Source: CAD feature listing. Evaluate the final solid. Frame: model axes, mm. Coordinates: 2 decimals unless noted, no trailing zeros. Order: outer loops, then holes, each group sorted by start corner. A loop starts at its lowest first (then second) coordinate and runs counter-clockwise, first axis right, second up.
Item 1: Mould query, pull axis Y, two halves, no side actions, for faces 1 (the flat face through (-41, 49, 1.6)), 2 (the cylindrical face through (5.533, 4.807, 0.789)), 3 (the cylindrical face through (-77.7, 84.3, 0.8)). Classes: released by +Y, released by -Y, zero draft, split by the parting line, or undercut.
Item 2: Section A-A on z = 1.05. Return the cut outline in (x, y), then the cut area to 3 significant figures.
Item 3: Ray query, line 1 (X direction, y = 8, z = 1.1); line 2 (Y direction, x = -2, z = 1.4); line 3 (Y direction, x = -69, z = 0.85). Return the intervals inside material, ascending.
Item 4: Section B-B on x = -70.5. Return the cut outline in (y, z), then the cut area to 3 significant figures.
Item 5: Contact query for flat-ended pins moving along their axis: P1, Ø0.8, axis at y = 91, z = 0.5, coming from the -X side; P2, Ø0.8, axis at x = -79, z = 0.5, coming from the +Y side. Output: stop coordinate, or through.
from build123d import *

# Parameters (mm, degrees)
BOSS_EXTRUDE1_DEPTH        = 1.6
F_3_2_3_2_DIAMETER_HOLE3_D = 3.2


with BuildPart() as part:
    # Sketch1 → Boss-Extrude1 (new body)
    with BuildSketch(Plane.XY):
        with BuildLine():
            Line((-87.56534388, 82.95185693), (-87.56534388, 6.95185693))
            ThreePointArc((-87.56534388, 6.95185693), (-86.686664224, 4.830536587), (-84.56534388, 3.95185693))
            Line((-84.56534388, 3.95185693), (3.43465612, 3.95185693))
            ThreePointArc((3.43465612, 3.95185693), (5.555976464, 4.830536587), (6.43465612, 6.95185693))
            Line((6.43465612, 6.95185693), (6.43465612, 88.95185693))
            ThreePointArc((6.43465612, 88.95185693), (5.555976464, 91.073177274), (3.43465612, 91.95185693))
            Line((3.43465612, 91.95185693), (0.93465612, 91.95185693))
            Line((0.93465612, 91.95185693), (-64.56534388, 91.95185693))
            Line((-64.56534388, 91.95185693), (-64.56534388, 87.95185693))
            ThreePointArc((-64.56534388, 87.95185693), (-65.151130318, 86.537643368), (-66.56534388, 85.95185693))
            Line((-66.56534388, 85.95185693), (-84.56534388, 85.95185693))
            ThreePointArc((-84.56534388, 85.95185693), (-86.686664224, 85.073177274), (-87.56534388, 82.95185693))
        make_face()
    extrude(amount=BOSS_EXTRUDE1_DEPTH)

    # Ø3.2 (3.2) Diameter Hole3 (through all)
    with Locations(Plane(origin=(0, 0, 0), x_dir=(-1, 0, 0), z_dir=(0, 0, -1))):
        with Locations((78.56534388, 6.95185693), (78.56534388, 82.95185693), (2.56534388, 82.95185693), (2.56534388, 6.95185693)):
            Hole(F_3_2_3_2_DIAMETER_HOLE3_D / 2)


solid = part.part
Answer list:
1. face 1: zero draft
1. face 2: released by -Y
1. face 3: undercut
2. outline: (-87.57, 6.95) arc R3 ccw to (-84.57, 3.95) - (3.43, 3.95) arc R3 ccw to (6.43, 6.95) - (6.43, 88.95) arc R3 ccw to (3.43, 91.95) - (-64.57, 91.95) - (-64.57, 87.95) arc R2 cw to (-66.57, 85.95) - (-84.57, 85.95) arc R3 ccw to (-87.57, 82.95) - close; hole circle Ø3.2 at (-78.57, 6.95); hole circle Ø3.2 at (-78.57, 82.95); hole circle Ø3.2 at (-2.57, 6.95); hole circle Ø3.2 at (-2.57, 82.95)
2. area: 8,090 mm2
3. line 1: x = -87.57 to -79.77, -77.36 to -3.77, -1.36 to 6.43
3. line 2: y = 3.95 to 5.46, 8.45 to 81.46, 84.45 to 91.95
3. line 3: y = 3.95 to 85.95
4. outline: (3.95, 0) - (85.95, 0) - (85.95, 1.6) - (3.95, 1.6) - close
4. area: 131 mm2
5. P1: stops at x = -64.57
5. P2: stops at y = 85.95
